Autodesk Inventor part; units mm, degrees
ref_plane "YZ Plane" through (0, 0, 0) normal (1, 0, 0) x (0, 1, 0)
ref_plane "XZ Plane" through (0, 0, 0) normal (0, 1, 0) x (-1, 0, 0)
ref_plane "XY Plane" through (0, 0, 0) normal (0, 0, 1) x (1, 0, 0)
sketch "Sketch1" plane through (0, 0, 0) normal (0, 1, 0) x (-1, 0, 0)
  circle A0 centre (0, 0) radius 26.1938
  circle A1 centre (0, 0) radius 18.2563
  dimension "d0" = 52.3875
  dimension "d1" = 36.5125
extrude "Extrusion1" add sketch "Sketch1" along normal blind 3.175
sketch "Sketch2" plane through (0, 0, 0) normal (0, 0, 1) x (1, 0, 0)
  line L0 (-22.225, 0) -> (-22.225, -1.5875)
  circle A0 centre (-22.225, -1.5875) radius 2.7781
  line L1 (0, 0) -> (0, 3.175)
  line L2 (26.1938, 3.175) -> (-26.1938, 3.175)
  dimension "d4" = 1.5875
  dimension "d5" = 5.5563
revolve "Revolution1" cut sketch "Sketch2" angle 360 about axis through (0, 0, 0) along (0, 1, 0)
chamfer "Chamfer1" distance 0.3969 angle 45 1 edges at (26.1938, 3.175, 0)
chamfer "Chamfer2" distance 0.3969 angle 45 1 edges at (26.1938, 0, 0)
chamfer "Chamfer3" distance 0.3969 angle 45 1 edges at (18.2563, 3.175, 0)
properties part number "ThrustBearing-LowerRing"
Could you check a few things on this model? Use its own coordinates, in mm. Coordinates: 2 decimals unless noted, no trailing zeros. Write each loop counter-clockwise with the first axis right and the second up, starting at its lowest first coordinate (ties: lowest second). Pieces come first, ordered by that corner, then holes. Notation, with made-up numbers: (75.5, 65) -> (124.5, 65) arc R21 ccw to (124.5, 89) -> close; hole circle Ø3 at (35.5, -19.5). An arc over 180 degrees is marked (long way). Write item = value, one per line. Start each with the question number.
(1) I need wall thicknesses on line 1 (X direction, y = 0.65, z = 11); line 2 (X direction, y = 0.3, z = 3.5); line 3 (Z direction, x = 0, y = 2.15). Which ranges of each line are inside material? Lowest first, please. Write a range as [from, to].
(2) I want a section at B-B (z = 0). Please give me the cut outline in (x, y) (1 decimal).
(3) We'd pull the mould along Z, two halves only. Please class faces 1 (the face through (-23, 0, -9)), 2 (the face through (3.41, 1.57, -25.97)), 3 (the face through (14.488, 1.37, 11.109)): released by +Z, released by -Z, zero draft, split by the parting line, or undercut.
(4) I want a section at A-A (x = 0). Please give me the cut outline in (y, z) (1 decimal).
(5) Will this pin go through, and if not, where does the flat tip stop? pin 1 (1.5 mm diameter, centred on x = -13.5, y = 2.5, fed in from -Z).
Result set:
q1.line_1 = [-23.77, -21.19], [-17.39, -14.57], [14.57, 17.39], [21.19, 23.77]
q1.line_2 = [-25.86, -24.01], [-19.88, -17.92], [17.92, 19.88], [24.01, 25.86]
q1.line_3 = [-26.19, -18.26], [18.26, 26.19]
q2.outline = (-26.2, 0.4) -> (-25.8, 0) -> (-24.5, 0) arc R2.8 cw to (-19.9, 0) -> (-18.3, 0) -> (-18.3, 2.8) -> (-18.7, 3.2) -> (-25.8, 3.2) -> (-26.2, 2.8) -> close; (18.3, 0) -> (19.9, 0) arc R2.8 cw to (24.5, 0) -> (25.8, 0) -> (26.2, 0.4) -> (26.2, 2.8) -> (25.8, 3.2) -> (18.7, 3.2) -> (18.3, 2.8) -> close
q3.face_1 = zero draft
q3.face_2 = split by the parting line
q3.face_3 = undercut
q4.outline = (0, -25.8) -> (0.4, -26.2) -> (2.8, -26.2) -> (3.2, -25.8) -> (3.2, -18.7) -> (2.8, -18.3) -> (0, -18.3) -> (0, -19.9) arc R2.8 cw to (0, -24.5) -> close; (0, 18.3) -> (2.8, 18.3) -> (3.2, 18.7) -> (3.2, 25.8) -> (2.8, 26.2) -> (0.4, 26.2) -> (0, 25.8) -> (0, 24.5) arc R2.8 cw to (0, 19.9) -> close
q5.pin_1 = -22.88
